Input: part model. Units: mm. Frame: model coordinates. Face numbers are marked on the shaded views. A direction names the side the tool comes from. Round coordinates to 2 decimals unless told otherwise and drop trailing zeros. Loops run counter-clockwise (first coordinate to the right, second up) from the corner with the lowest first, then second, coordinate; pieces in that order, holes last. Notation, with made-up numbers: M 60,87 L 64,87 A20 ccw 64,109 Z; hole C 46,70.25 d9. An arc over 180 degrees is marked long. Put each result on its own line as item: value. Start each with the question number.
1) Section D-D on x = -18.5. Output: boundary loops of the cut face in (y, z).
2) Reachability of the marked faces 5 and 6 from +Z, -Z, +X, -X, +Y, -Y: full face, straight path, thin tool, end or side. Return the list, or none.
3) Pin query (flat end, axial travel): pin 1 (1.5 mm diameter, centred on x = 5, z = 18, fed in from -Y); pin 2 (10 mm diameter, centred on x = 8, y = 18, fed in from +Z); pin 3 (2 mm diameter, centred on x = -19, y = 1.5, fed in from -Z); pin 4 (1.5 mm diameter, centred on x = 17, y = 21, fed in from -Z). Return the tip coordinate at first contact, or that it passes through.
4) Section B-B on x = 6.5. Output: boundary loops of the cut face in (y, z), plus the area to 3 significant figures.
5) Line query: probe 1 along X at (y, z) = (9, 12.75); probe 2 along Y at (x, z) = (17.5, 13); probe 3 along Y at (x, z) = (-17.5, 15). Output: solid intervals per line, ascending.
6) Draft query along X for the marked faces 1, 2, 3 and 4. Return one class per face: +X half, -X half, draft (parallel to the pull), parting line (faces both ways), or undercut.
7) Section C-C on z = 16. Output: boundary loops of the cut face in (x, y), plus the area to 3 significant figures.
8) Section A-A on y = 10.5. Output: boundary loops of the cut face in (x, z).
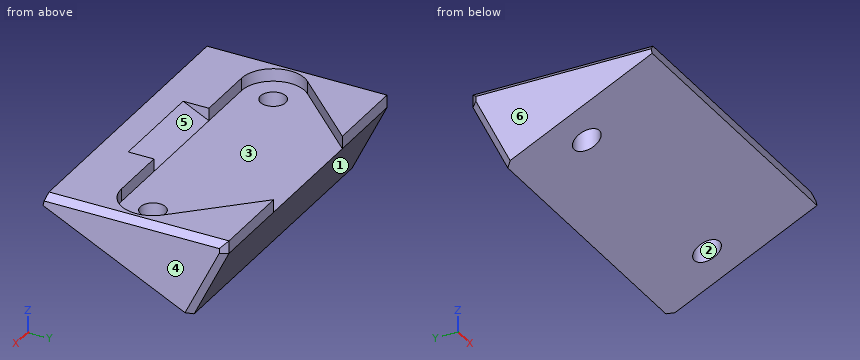
from build123d import *

# Parameters (mm, degrees)
SKETCH_W        = 48
SKETCH_H        = 48
PAD_DEPTH       = 20
POCKET_DEPTH    = 2
POCKET001_DEPTH = 48.001
SKETCH003_R     = 2
POCKET002_DEPTH = 11.221735
CHAMFER_SIZE    = 1
CHAMFER001_SIZE = 4
POCKET003_DEPTH = 16


with BuildPart() as part:
    # Sketch → Pad (new body)
    with BuildSketch(Plane.XY):
        Rectangle(SKETCH_W, SKETCH_H)
    extrude(amount=PAD_DEPTH)

    # Sketch001 (on Face6 of Pad) → Pocket (cut)
    with BuildSketch(Plane.XY.offset(20)):
        with BuildLine():
            Line((-10, 24), (10, 24))
            Line((10, 24), (21.102083, 12.467708))
            ThreePointArc((17.5, 4), (22.101008, 7.042775), (21.102083, 12.467708))
            Line((-17.5, 4), (17.5, 4))
            ThreePointArc((-21.102083, 12.467708), (-22.101008, 7.042775), (-17.5, 4))
            Line((-10, 24), (-21.102083, 12.467708))
        make_face()
    extrude(amount=-POCKET_DEPTH, mode=Mode.SUBTRACT)

    # Sketch002 (on Face9 of Pocket) → Pocket001 (cut, through all)
    with BuildSketch(Plane.YZ.offset(24)):
        Polygon((-8.438403, 20), (18.49136, 6.779265), (24, 18), (24, 0), (-24, 0), (-24, 20), align=None)
    extrude(amount=-POCKET001_DEPTH, mode=Mode.SUBTRACT)

    # Sketch003 (on Face8 of Pocket001) → Pocket002 (cut, through all)
    with BuildSketch(Plane.XY.offset(18)):
        with Locations((-17.5, 9)):
            Circle(SKETCH003_R)
        with Locations((17.5, 9)):
            Circle(SKETCH003_R)
    extrude(amount=-POCKET002_DEPTH, mode=Mode.SUBTRACT)

    # Chamfer
    chamfer_edges = [part.edges().sort_by_distance(p)[0] for p in [
        (24, 7.780798, 20),
        (24, 24, 19),
        (24, 21.24568, 12.389633),
        (-24, 21.24568, 12.389633),
        (-24, 24, 19),
        (-24, 7.780798, 20),
    ]]
    chamfer(chamfer_edges, length=CHAMFER_SIZE)

    # Chamfer001
    chamfer001_edges = [part.edges().sort_by_distance(p)[0] for p in [
        (0, -8.438403, 20),
    ]]
    chamfer(chamfer001_edges, length=CHAMFER001_SIZE)

    # Sketch004 (on Face7 of Chamfer001) → Pocket003 (cut)
    with BuildSketch(Plane.YZ.offset(8)):
        Polygon((4, 18), (-0.073868, 20), (4, 20), align=None)
    extrude(amount=-POCKET003_DEPTH, mode=Mode.SUBTRACT)


solid = part.part
Geometry results:
1. outline: M -4.85,18.24 L 7.27,12.29 L 7.27,18 L 4.1,18 L 4.1,20 L -4.44,20 Z; M 10.73,10.59 L 18.49,6.78 L 24,18 L 24,20 L 15.17,20 L 15.17,18 L 10.73,18 Z
2. face 5: +Z, +Y
2. face 6: +Z, -Z, -X, +Y, -Y
3. pin 1: stops at y = -4.85
3. pin 2: stops at z = 18
3. pin 3: stops at z = 14.63
3. pin 4: stops at z = 10.36
4. outline: M -4.85,18.24 L 18.49,6.78 L 24,18 L 4,18 L -0.07,20 L -4.44,20 Z
4. area: 172 mm²
5. probe 1: x = -24 to -19.5, -15.5 to 15.5, 19.5 to 24
5. probe 2: y = 5.82 to 7, 11 to 21.55
5. probe 3: y = 1.75 to 7, 11 to 22.53
6. face 1: draft
6. face 2: undercut
6. face 3: undercut
6. face 4: +X half
7. outline: M -24,-0.29 L 24,-0.29 L 24,21.9 L 23,23.02 L -23,23.02 L -24,21.9 Z; hole C -17.5,9 d4; hole C 17.5,9 d4
7. area: 1,090 mm²
8. outline: M -24,10.7 L -18.82,10.7 L -18.82,18 L -22.27,18 L -22.27,20 L -23,20 L -24,19 Z; M -16.18,10.7 L 16.18,10.7 L 16.18,18 L -16.18,18 Z; M 18.82,10.7 L 24,10.7 L 24,19 L 23,20 L 22.27,20 L 22.27,18 L 18.82,18 Z
